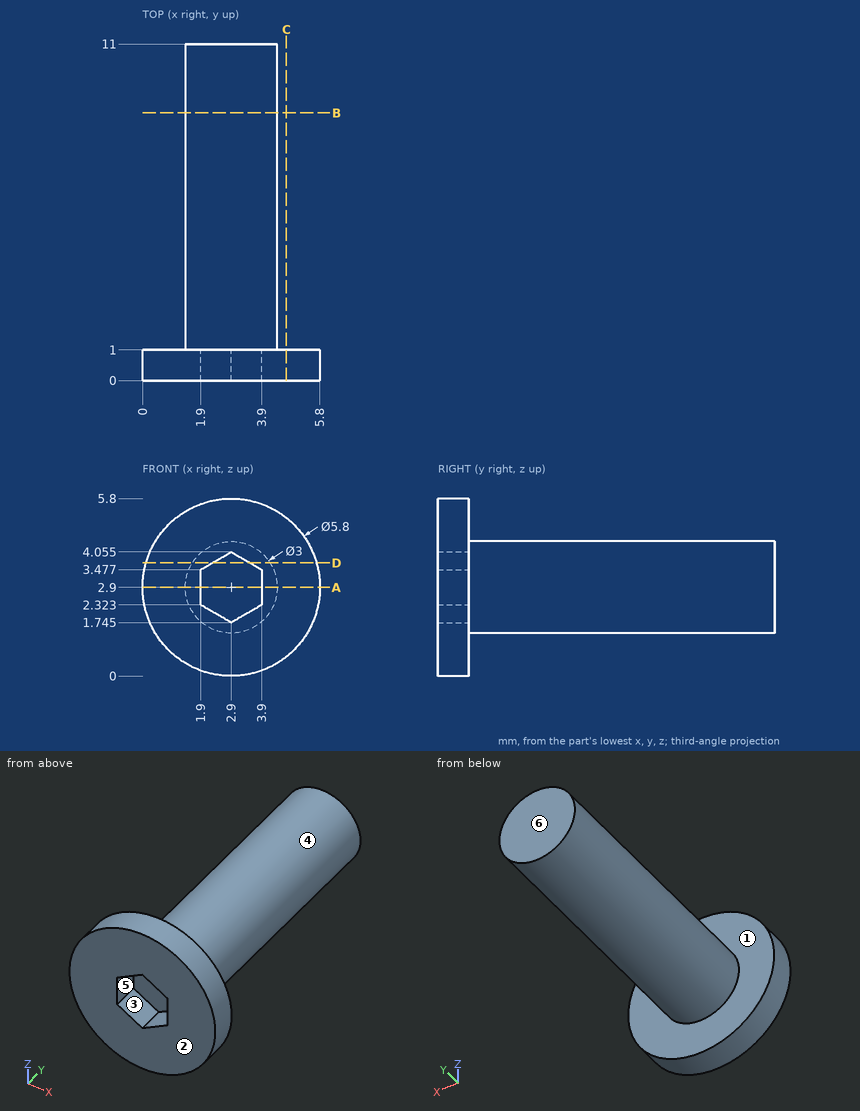
Could you check a few things on this drawing? It's one solid part, dimensions in mm from its lowest x, y, z. A direction names the side the tool comes from. Round coordinates to 2 decimals unless told otherwise and drop trailing zeros. Loops run counter-clockwise (first coordinate to the right, second up) from the corner with the lowest first, then second, coordinate; pieces in that order, holes last. Notation, with made-up numbers: M 34,35.25 L 83,35.25 A24 cw 83,57.25 Z; hole C -18,-2.5 d4. An arc over 180 degrees is marked long. Write item = value, one per line. Start each with the question number.
(1) If we mould it in two halves opening along Z, with no side actions, what happens to the marked faces 3, 4, 5 and 6? For each: released by +Z, released by -Z, zero draft, split by the parting line, or undercut.
(2) I need wall thicknesses on line 1 along Y through (x, z) = (3.85, 0.4); line 2 along X through (y, z) = (0.5, 1.8) (1 decimal); line 3 along Z through (x, y) = (0.35, 0.75). Which ranges of each line are inside material? Lowest first, please.
(3) Suppose I cut it at D-D on z = 3.7. Write out the boundary of the cut face in (x, y) (1 decimal).
(4) I'm going to push a flat-ended pin straight in: P1, Ø0.6, axis at x = 3, z = 3, coming from the -Y side. Where does the tip first touch, or does it pass through?
(5) Suppose I cut it at B-B on y = 8.75. Write out the boundary of the cut face in (x, z).
(6) Suppose I cut it at A-A on z = 2.9. Write out the boundary of the cut face in (x, y), plus the area to 3 significant figures.
(7) Which directions (+Z, -Z, +X, -X, +Y, -Y) give clear straight access to the entire face, cutting with the end or side of a thin tool? Please do the marked faces 1 and 2.
(8) Suppose I cut it at C-C on x = 4.7. Write out the boundary of the cut face in (y, z).
Answer block:
q1.face_3 = undercut
q1.face_4 = split by the parting line
q1.face_5 = undercut
q1.face_6 = zero draft
q2.line_1 = 0 to 1
q2.line_2 = 0.2 to 2.8, 3 to 5.6
q2.line_3 = 1.52 to 4.28
q3.outline = M 0.1,0 L 2.3,0 L 2.3,1 L 3.5,1 L 3.5,0 L 5.7,0 L 5.7,1 L 4.2,1 L 4.2,11 L 1.6,11 L 1.6,1 L 0.1,1 Z
q4.P1 = 1
q5.outline = C 2.9,2.9 d3
q6.outline = M 0,0 L 1.9,0 L 1.9,1 L 3.9,1 L 3.9,0 L 5.8,0 L 5.8,1 L 4.4,1 L 4.4,11 L 1.4,11 L 1.4,1 L 0,1 Z
q6.area = 33.8 mm²
q7.face_1 = +Y
q7.face_2 = +Z, -Z, +X, -X, -Y
q8.outline = M 0,0.63 L 1,0.63 L 1,5.17 L 0,5.17 Z
